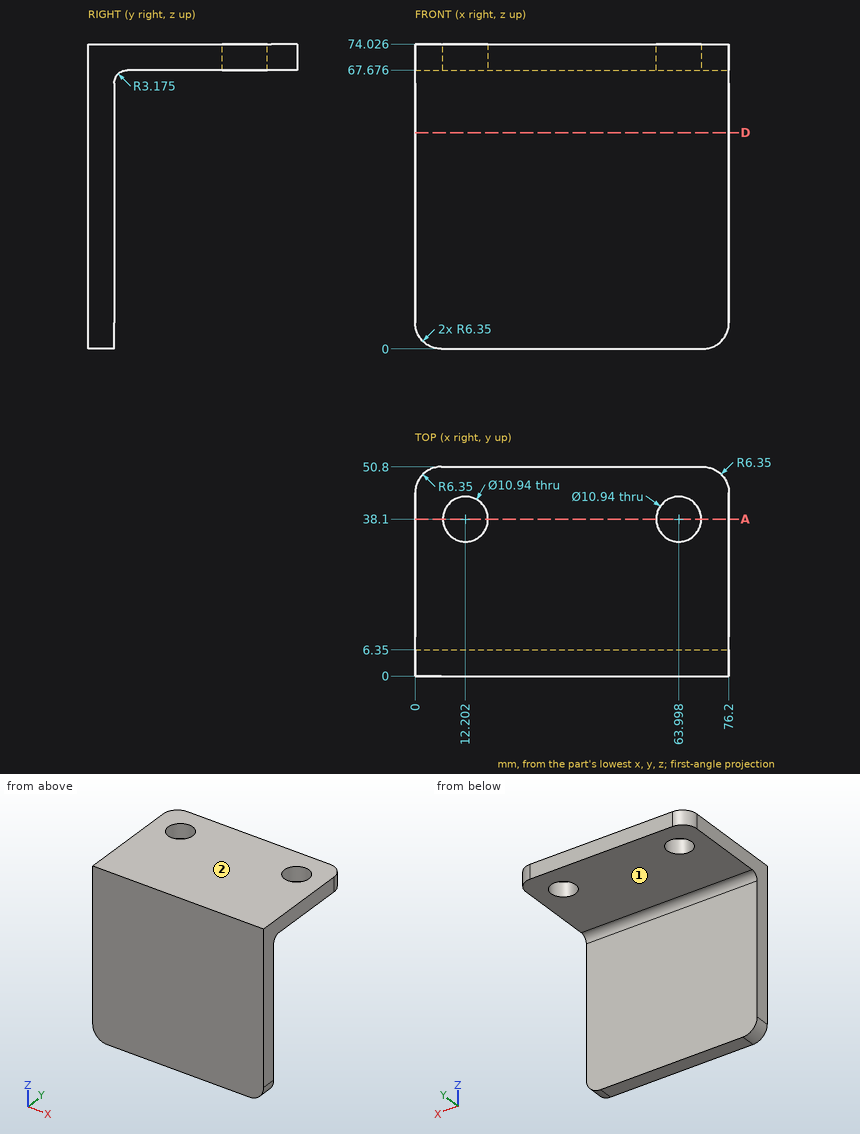
Geometry check sheet. Reference: drawing and pictorial views, mm from the part's lowest x, y, z. A direction names the side the tool comes from. Coordinates: 2 decimals unless noted, no trailing zeros. Order: outer loops, then holes, each group sorted by start corner. A loop starts at its lowest first (then second) coordinate and runs counter-clockwise, first axis right, second up. Notation, with made-up numbers: (6, -25) -> (50, -25) arc R11 ccw to (50, -14) -> close; hole circle Ø3 at (-9.75, 9.5). An arc over 180 degrees is marked (long way). Use CSV: the item, a comma, the result in double quotes. Start each with the question number.
Q1. Thickness scan on line 1 along X through (y, z) = (38, 72); line 2 along Y through (x, z) = (38, 46.5); line 3 along Z through (x, y) = (44, 45.5). Record the ranges inside material, lowest first.
Q2. Section check D-D, the plane z = 52.5. Record the cut outline in (x, y).
Q3. Depth check by flat-ended pin: P1, Ø2, axis at x = 16, y = 45, coming from the -Z side; P2, Ø1.5, axis at x = 26.5, z = 9.5, coming from the +Y side; P3, Ø10, axis at x = 64, y = 38.1, coming from the +Z side. Enter the tip coordinate at first touch or a pass-through.
Q4. Tool access check on the marked faces 1 and 2. Record the directions out of +Z, -Z, +X, -X, +Y, -Y that give a thin tool (end or side, any length) a straight path to the whole face; none if there is none.
Q5. Section check A-A, the plane y = 38.1. Record the cut outline in (x, z).
Returned:
1,line 1,"x = 0 to 6.73, 17.67 to 58.53, 69.47 to 76.2"
1,line 2,"y = 0 to 6.35"
1,line 3,"z = 67.68 to 74.03"
2,outline,"(0, 0) -> (76.2, 0) -> (76.2, 6.35) -> (0, 6.35) -> close"
3,P1,"stops at z = 67.68"
3,P2,"stops at y = 6.35"
3,P3,"passes through"
4,face 1,"-Z, +X, -X, +Y"
4,face 2,"+Z, +X, -X, +Y, -Y"
5,outline,"(0, 67.68) -> (6.73, 67.68) -> (6.73, 74.03) -> (0, 74.03) -> close; (17.67, 67.68) -> (58.53, 67.68) -> (58.53, 74.03) -> (17.67, 74.03) -> close; (69.47, 67.68) -> (76.2, 67.68) -> (76.2, 74.03) -> (69.47, 74.03) -> close"
